Model file for the job. Use its own axes, mm. Give positions to 0.01 mm unless a question says otherwise; leave off trailing zeros. Write each loop counter-clockwise with the first axis right and the second up, starting at its lowest first coordinate (ties: lowest second). Pieces come first, ordered by that corner, then holes. Notation, with made-up numbers: M -16.75,24 L 9.25,24 A26 cw 9.25,49 Z; hole C -8.5,-31 d9. An arc over 180 degrees is marked long. Answer as a JSON object with one key per item and string values. Group by question number.
```python
from build123d import *

# Parameters (mm, degrees)
F0_R     = 1.7272
F0_R_2   = 3.96875
F0_R_3   = 10.31875
F0_R_4   = 11.1125
F1_DEPTH = 3.175
F3_DEPTH = 3.175
F4_COUNT = 6
F4_ANGLE = 300
F5_R     = 11.1125
F6_DEPTH = 1.94945


with BuildPart() as f1:
    # F0 (on Top) → F1 (new body)
    with BuildSketch(Plane.XY):
        with BuildLine():
            Line((-447.0158774883, 32.54375), (-488.3522532774, 21.4677014893))
            ThreePointArc((-488.3522532774, 21.4677014893), (-504.825, 0), (-488.3522532774, -21.4677014893))
            Line((-488.3522532774, -21.4677014893), (-447.0158774883, -32.54375))
            Line((-447.0158774883, -32.54375), (-440.6658774883, -32.54375))
            Line((-440.6658774883, -32.54375), (-440.6658774883, -29.36875))
            Line((-440.6658774883, -29.36875), (-41.9341225117, -29.36875))
            Line((-41.9341225117, -29.36875), (-41.9341225117, -32.54375))
            Line((-41.9341225117, -32.54375), (-35.5841225117, -32.54375))
            Line((-35.5841225117, -32.54375), (5.7522532774, -21.4677014893))
            ThreePointArc((5.7522532774, -21.4677014893), (22.225, 0), (5.7522532774, 21.4677014893))
            Line((5.7522532774, 21.4677014893), (-35.5841225117, 32.54375))
            Line((-35.5841225117, 32.54375), (-41.9341225117, 32.54375))
            Line((-41.9341225117, 32.54375), (-41.9341225117, 29.36875))
            Line((-41.9341225117, 29.36875), (-440.6658774883, 29.36875))
            Line((-440.6658774883, 29.36875), (-440.6658774883, 32.54375))
            Line((-440.6658774883, 32.54375), (-447.0158774883, 32.54375))
        make_face()
        with Locations((-426.3783774883, -24.60625)):
            Circle(F0_R, mode=Mode.SUBTRACT)
        with Locations((-494.3865861589, -11.7865861589)):
            Circle(F0_R, mode=Mode.SUBTRACT)
        with Locations((-470.8134138411, -11.7865861589)):
            Circle(F0_R_2, mode=Mode.SUBTRACT)
        with Locations((-56.2216225117, -24.60625)):
            Circle(F0_R, mode=Mode.SUBTRACT)
        with Locations((-11.7865861589, -11.7865861589)):
            Circle(F0_R_2, mode=Mode.SUBTRACT)
        with Locations((11.7865861589, -11.7865861589)):
            Circle(F0_R, mode=Mode.SUBTRACT)
        with Locations((-482.6, 0)):
            Circle(F0_R_3, mode=Mode.SUBTRACT)
        with Locations((-494.3865861589, 11.7865861589)):
            Circle(F0_R_2, mode=Mode.SUBTRACT)
        with Locations((-470.8134138411, 11.7865861589)):
            Circle(F0_R, mode=Mode.SUBTRACT)
        with Locations((-426.3783774883, 24.60625)):
            Circle(F0_R, mode=Mode.SUBTRACT)
        Circle(F0_R_4, mode=Mode.SUBTRACT)
        with Locations((-11.7865861589, 11.7865861589)):
            Circle(F0_R, mode=Mode.SUBTRACT)
        with Locations((11.7865861589, 11.7865861589)):
            Circle(F0_R_2, mode=Mode.SUBTRACT)
        with Locations((-56.2216225117, 24.60625)):
            Circle(F0_R, mode=Mode.SUBTRACT)
    extrude(amount=F1_DEPTH)

    # F2 (on face) → F3 (cut, through all)
    with BuildSketch(Plane(origin=(0, 0, 0), x_dir=(1, 0, 0), z_dir=(0, 0, -1))):
        with BuildLine():
            ThreePointArc((-489.8964580984, -7.2964580984), (-491.5362996353, -5.159375), (-492.56714712, -2.6706890217))
            Line((-492.56714712, -2.6706890217), (-494.1005543693, -3.0815642558))
            ThreePointArc((-494.1005543693, -3.0815642558), (-492.9111149638, -5.953125), (-491.0189901135, -8.4189901135))
            Line((-491.0189901135, -8.4189901135), (-489.8964580984, -7.2964580984))
        make_face()
    f3 = extrude(amount=-F3_DEPTH, mode=Mode.SUBTRACT)

    # F4: F3 ×6 about axis
    f4_axis = Axis((-482.6, 0, 0), (0, 0, -1))
    for i in range(1, F4_COUNT):
        add(f3.rotate(f4_axis, i * F4_ANGLE / (F4_COUNT - 1)), mode=Mode.SUBTRACT)

    # F5 (on face) → F6 (cut)
    with BuildSketch(Plane(origin=(0, 0, 0), x_dir=(1, 0, 0), z_dir=(0, 0, -1))):
        with Locations((-482.6, 0)):
            Circle(F5_R)
    extrude(amount=-F6_DEPTH, mode=Mode.SUBTRACT)


solid = f1.part
```
Q1. Slice it at A-A, the plane x = 0. Write the cut outline in (y, z) (1 decimal), then the cut area to 3 significant figures.
Q2. Wall check: L1, parallel to X at y = 14, z = 1.85; L2, parallel to X at y = -15, z = 0.6; L3, parallel to Y at x = -329.5, z = 0.6. Give the ranges that are in metal, low to high.
Q3. Slice it at B-B, the plane x = -155.5. Write the cut outline in (y, z) (3 decimals), then the cut area to 3 significant figures.
Q4. Two-plate mould, pull along Y, no slides. Class faces 1 (the flat face through (-15.205, -27.083, 1.565)), 2 (the cylindrical face through (10.6, 3.34, 1.57)), 3 (the flat face through (-245, 0, 0)), 4 (the flat face through (-467.395, 27.083, 1.565)): +Y half, -Y half, draft (parallel to the pull), parting line (faces both ways), or undercut.
Q5. Drop flat-ended pins along their axis: P1, Ø1.6, axis at x = -182, z = 2, coming from the +Y side; P2, Ø1.6, axis at x = -274.5, z = 2, coming from the -Y side; P3, Ø1.7, axis at x = -477, y = -8, coming from the -Z side. Give the stop position or say it passes through.
Solved:
{
 "1": {"outline": "M -23,0 L -11.1,0 L -11.1,3.2 L -23,3.2 Z; M 11.1,0 L 23,0 L 23,3.2 L 11.1,3.2 Z", "area": "75.5 mm²"},
 "2": {"L1": "x = -499.86 to -497.68, -491.09 to 8.49, 15.08 to 17.26", "L2": "x = -499 to -473.14, -468.48 to -14.12, -9.46 to 16.4", "L3": "y = -29.37 to 29.37"},
 "3": {"outline": "M -29.369,0 L 29.369,0 L 29.369,3.175 L -29.369,3.175 Z", "area": "186 mm²"},
 "4": {"face 1": "-Y half", "face 2": "undercut", "face 3": "draft", "face 4": "+Y half"},
 "5": {"P1": "stops at y = 29.37", "P2": "stops at y = -29.37", "P3": "stops at z = 1.95"}
}
